Build history of the part. All positions in model axes, mm. Face numbers are marked on the shaded views. A direction names the side the tool comes from. Give positions to 0.01 mm unless a question says otherwise; leave off trailing zeros. Loops run counter-clockwise (first coordinate to the right, second up) from the corner with the lowest first, then second, coordinate; pieces in that order, holes last. Notation, with made-up numbers: (23, -25.75) -> (34, -25.75) arc R27 cw to (34, -5.75) -> close; hole circle Ø2 at (67, 82). An arc over 180 degrees is marked (long way). Answer in a Markdown table with one row per item. Add a question column.
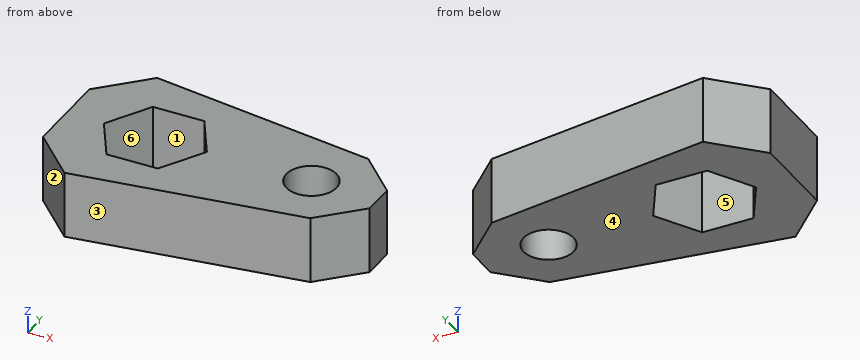
Autodesk Inventor part; units mm, degrees
ref_plane "YZ Plane" through (0, 0, 0) normal (1, 0, 0) x (0, 1, 0)
ref_plane "XZ Plane" through (0, 0, 0) normal (0, 1, 0) x (-1, 0, 0)
ref_plane "XY Plane" through (0, 0, 0) normal (0, 0, 1) x (1, 0, 0)
sketch "Sketch1" plane through (0, 0, 0) normal (0, 0, 1) x (1, 0, 0)
  line L0 (-4, -8) -> (16.5, -5)
  line L1 (20, -1.5) -> (20, 1.5)
  line L2 (16.5, 5) -> (-4, 8)
  line L3 (-8, 4) -> (-8, -4)
  line L4 (-4, 8) -> (-8, 4)
  line L5 (-8, -4) -> (-4, -8)
  line L6 (16.5, -5) -> (20, -1.5)
  line L7 (20, 1.5) -> (16.5, 5)
  circle A0 centre (0, 0) radius 2.75
  circle A1 centre (14, 0) radius 2.25
  circle A2 centre (0, 0) radius 5 construction
  circle A3 centre (14, 0) radius 4.5 construction
  point P0 (-8, 0)
  point P1 (20, 0)
  dimension "d9" = 8
  dimension "d10" = 14
  dimension "d11" = 4.5
  dimension "d12" = 5.5
  dimension "d13" = 6
  dimension "d16" = 10
  dimension "d17" = 9
  dimension "d18" = 8
  dimension "d19" = 4
  dimension "d20" = 4
  dimension "d21" = 4
  dimension "d22" = 10
  dimension "d23" = 3
extrude "Extrusion1" add sketch "Sketch1" along normal blind 6
sketch "Sketch2" plane through (0, 0, 6) normal (0, 0, 1) x (1, 0, 0)
  circle A0 centre (0, 0) radius 2.75
  line L0 (-8, 4) -> (-8, -4)
  line L1 (4.6188, 0) -> (2.3094, -4)
  line L2 (2.3094, -4) -> (-2.3094, -4)
  line L3 (-2.3094, -4) -> (-4.6188, 0)
  line L4 (-4.6188, 0) -> (-2.3094, 4)
  line L5 (-2.3094, 4) -> (2.3094, 4)
  line L6 (2.3094, 4) -> (4.6188, 0)
  dimension "d24" = 8
extrude "Extrusion2" cut sketch "Sketch2" against normal blind 6
properties part number "y_carriage_nut_holder_a"
(1) Saw through at B-B, the plane z = 2.1. List the corners of the cut face in (x, y).
(2) Two-plate mould, pull along X, no slides. Class the marked faces 3, 4, 5 and 6: released by +X, released by -X, zero draft, split by the parting line, or undercut.
(3) Wall check: line 1 along X through (y, z) = (-1.75, 4.5); line 2 along X through (y, z) = (-3, 3.15); line 3 along X through (y, z) = (-2, 5.6). Give the ranges that are in metal, low to high. Write a range as from..to.
(4) Saw through at D-D, the plane x = 10.5. List the corners of the cut face in (y, z).
(5) 3-axis set-ups, long thin cutter, end or side, ignore diameter. For the marked faces 1 and 2: which of +Z, -Z, +X, -X, +Y, -Y reach the whole face in a straight line?
(6) Saw through at C-C, the plane x = -1. List the corners of the cut face in (y, z), then the cut area to 3 significant figures.
(7) Flat gauge pins, fed straight in: pin 1 Ø1.5 at (x, z) = (1.5, 3.5) entering from +Y; pin 2 Ø3 at (x, z) = (8, 1) entering from +Y; pin 3 Ø1.4 at (x, z) = (0.5, 4.5) entering from +Y; pin 4 Ø3.5 at (x, y) = (14, 0) entering from +Z. Where does each tip first touch, or does it go through?
(8) Saw through at A-A, the plane x = 3. List the corners of the cut face in (y, z).
Worked answers:
| question | item | result |
|---|---|---|
| 1 | outline | (-8, -4) -> (-4, -8) -> (16.5, -5) -> (20, -1.5) -> (20, 1.5) -> (16.5, 5) -> (-4, 8) -> (-8, 4) -> close; hole (-4.62, 0) -> (-2.31, -4) -> (2.31, -4) -> (4.62, 0) -> (2.31, 4) -> (-2.31, 4) -> close; hole circle Ø4.5 at (14, 0) |
| 2 | face 3 | released by +X |
| 2 | face 4 | zero draft |
| 2 | face 5 | undercut |
| 2 | face 6 | undercut |
| 3 | line 1 | -8..-3.61, 3.61..12.59, 15.41..19.75 |
| 3 | line 2 | -8..-2.89, 2.89..18.5 |
| 3 | line 3 | -8..-3.46, 3.46..12.97, 15.03..19.5 |
| 4 | outline | (-5.88, 0) -> (5.88, 0) -> (5.88, 6) -> (-5.88, 6) -> close |
| 5 | face 1 | +Z, -Z |
| 5 | face 2 | +Z, -Z, -X, -Y |
| 6 | outline | (-7.56, 0) -> (-4, 0) -> (-4, 6) -> (-7.56, 6) -> close; (4, 0) -> (7.56, 0) -> (7.56, 6) -> (4, 6) -> close |
| 6 | area | 42.7 mm^2 |
| 7 | pin 1 | y = 7.3 |
| 7 | pin 2 | y = 6.46 |
| 7 | pin 3 | y = 7.44 |
| 7 | pin 4 | through |
| 8 | outline | (-6.98, 0) -> (-2.8, 0) -> (-2.8, 6) -> (-6.98, 6) -> close; (2.8, 0) -> (6.98, 0) -> (6.98, 6) -> (2.8, 6) -> close |
